```python
from build123d import *

# Parameters (mm, degrees)
CROQUIS1_R                 = 4
SALIENTE_EXTRUIR1_DEPTH    = 12.5
CROQUIS2_W                 = 30
CROQUIS2_H                 = 15
CORTAR_EXTRUIR1_DEPTH      = 52.973550966
CROQUIS3_R                 = 4
CORTAR_EXTRUIR2_DEPTH      = 52.973550966
CROQUIS4_R                 = 11.25
CORTAR_EXTRUIR3_DEPTH      = 3.5
CORTAR_EXTRUIR4_DEPTH      = 52.278650528
CORTAR_EXTRUIR4_DEPTH_BACK = 52.278650528
CROQUIS5_R                 = 5.25
CROQUIS6_R                 = 16.25
CROQUIS6_R_2               = 11.25
SALIENTE_EXTRUIR2_DEPTH    = 12
CHAFL_N1_SIZE              = 1
SKETCH1_R                  = 1.75
CUT_EXTRUDE1_DEPTH         = 10
CIRPATTERN1_COUNT          = 4


with BuildPart() as part:
    # Croquis1 → Saliente-Extruir1 (new, symmetric)
    with BuildSketch(Plane.XY):
        with BuildLine():
            Line((-43, 6), (43, 6))
            ThreePointArc((43, 6), (49, 0), (43, -6))
            Line((43, -6), (-43, -6))
            ThreePointArc((-43, -6), (-49, 0), (-43, 6))
        make_face()
        with Locations((-43, 0)):
            Circle(CROQUIS1_R, mode=Mode.SUBTRACT)
        with Locations((43, 0)):
            Circle(CROQUIS1_R, mode=Mode.SUBTRACT)
    extrude(amount=SALIENTE_EXTRUIR1_DEPTH, both=True)

    # Croquis2 → Cortar-Extruir1 (cut, through all)
    with BuildSketch(Plane(origin=(0, 6, 0), x_dir=(1, 0, 0), z_dir=(0, 1, 0))):
        with Locations((-34, 0)):
            Rectangle(CROQUIS2_W, CROQUIS2_H)
        with Locations((34, 0)):
            Rectangle(CROQUIS2_W, CROQUIS2_H)
    extrude(amount=-CORTAR_EXTRUIR1_DEPTH, mode=Mode.SUBTRACT)

    # Croquis3 → Cortar-Extruir2 (cut, through all)
    with BuildSketch(Plane(origin=(0, 6, 0), x_dir=(1, 0, 0), z_dir=(0, 1, 0))):
        with Locations(Location((0, 0, 0), (0, 0, 270))):
            Circle(CROQUIS3_R)
    extrude(amount=-CORTAR_EXTRUIR2_DEPTH, mode=Mode.SUBTRACT)

    # Croquis4 → Cortar-Extruir3 (cut)
    with BuildSketch(Plane(origin=(0, 6, 0), x_dir=(1, 0, 0), z_dir=(0, 1, 0))):
        with Locations(Location((0, 0, 0), (0, 0, 270))):
            Circle(CROQUIS4_R)
    extrude(amount=-CORTAR_EXTRUIR3_DEPTH, mode=Mode.SUBTRACT)

    # Croquis5 → Cortar-Extruir4 (cut, two sides: drawn at the far end of the back side and taken through both)
    with BuildSketch(Plane(origin=(0, 2.5, 0), x_dir=(1, 0, 0), z_dir=(0, 1, 0)).offset(-CORTAR_EXTRUIR4_DEPTH_BACK)):
        with Locations(Location((0, 0, 0), (0, 0, 270))):
            Circle(CROQUIS5_R)
    extrude(amount=CORTAR_EXTRUIR4_DEPTH + CORTAR_EXTRUIR4_DEPTH_BACK, mode=Mode.SUBTRACT)

    # Croquis6 → Saliente-Extruir2 (add)
    with BuildSketch(Plane(origin=(0, 6, 0), x_dir=(1, 0, 0), z_dir=(0, 1, 0))):
        Circle(CROQUIS6_R)
        with Locations(Location((0, 0, 0), (0, 0, 270))):
            Circle(CROQUIS6_R_2, mode=Mode.SUBTRACT)
    extrude(amount=-SALIENTE_EXTRUIR2_DEPTH)

    # Chaflán1
    chafl_n1_edges = [part.edges().sort_by_distance(p)[0] for p in [
        (0, -6, -16.25),
        (0, 6, -16.25),
        (0, 6, 16.25),
        (0, -6, 16.25),
        (49, 0, 12.5),
        (26.691639914, 6, 12.5),
        (-49, 0, -7.5),
        (-31, -6, -7.5),
        (-49, 0, 7.5),
        (-31, -6, 7.5),
        (-19, 0, 7.5),
        (-19, -6, 0),
        (-31, 6, 7.5),
        (-19, 6, 0),
        (-31, 6, -7.5),
        (-49, 0, 12.5),
        (26.691639914, 6, -12.5),
        (31, 6, 7.5),
        (31, 6, -7.5),
        (19, 6, 0),
        (49, 0, -7.5),
        (31, -6, -7.5),
        (49, 0, 7.5),
        (31, -6, 7.5),
        (49, 0, -12.5),
        (19, -6, 0),
        (-26.691639914, -6, -12.5),
        (-49, 0, -12.5),
        (-26.691639914, -6, 12.5),
        (-26.691639914, 6, 12.5),
        (-26.691639914, 6, -12.5),
        (26.691639914, -6, -12.5),
        (26.691639914, -6, 12.5),
    ]]
    chamfer(chafl_n1_edges, length=CHAFL_N1_SIZE)

    # Sketch1 → Cut-Extrude1 (cut)
    with BuildSketch(Plane(origin=(0, 2.5, 0), x_dir=(1, 0, 0), z_dir=(0, 1, 0))):
        with Locations(Location((0, 8, 0), (0, 0, 270))):
            Circle(SKETCH1_R)
    cut_extrude1 = extrude(amount=-CUT_EXTRUDE1_DEPTH, mode=Mode.SUBTRACT)

    # CirPattern1: Cut-Extrude1 ×4 about axis
    cirpattern1_axis = Axis((0, 0, 0), (0, 1, 0))
    for i in range(1, CIRPATTERN1_COUNT):
        add(cut_extrude1.rotate(cirpattern1_axis, i * 360 / CIRPATTERN1_COUNT), mode=Mode.SUBTRACT)


solid = part.part
```
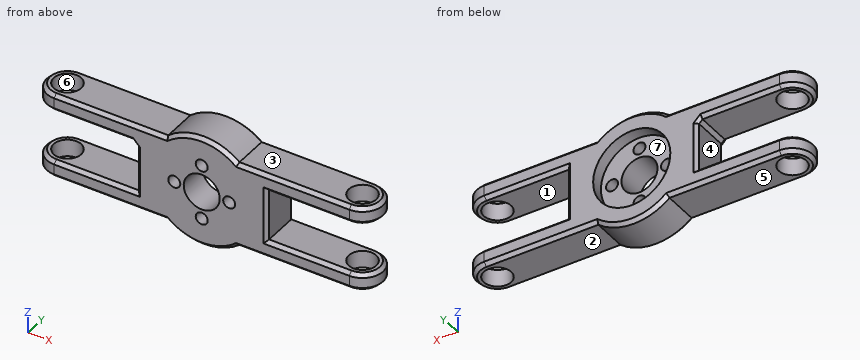
For this review, take the finished solid that the model builds, in its own axes (mm). Face numbers are marked on the shaded views. A direction names the side the tool comes from. Round coordinates to 2 decimals unless told otherwise and drop trailing zeros. Write each loop counter-clockwise with the first axis right and the second up, starting at its lowest first coordinate (ties: lowest second). Pieces come first, ordered by that corner, then holes. Notation, with made-up numbers: (-6, 30.25) - (9, 30.25) arc R5 cw to (9, 38.25) - close; hole circle Ø5 at (34.5, 21.25). An arc over 180 degrees is marked (long way). Answer as a JSON object with one key per item and string values.
1. We need section B-B on y = 0. Count the separate pieces of the cut face and the enclosed holes in it, then the cut area to 3 significant figures.
Response values:
{"separate pieces": "5", "enclosed holes": "5", "area": "1,370 mm2"}
2. For pin 1 Ø5 at (x, y) = (-34.5, 2) entering from +Z; pin 2 Ø4.5 at (x, z) = (-8, 0) entering from +Y; pin 3 Ø1.5 at (y, z) = (-0.5, 4) entering from -X, all flat-tipped, find the tip position at first contact; note any pin that passes through.
Response values:
{"pin 1": "stops at z = 12.5", "pin 2": "stops at y = 2.5", "pin 3": "stops at x = -19"}
3. We need section C-C on x = -15. Give the boundary of the cut face in (y, z), then the cut area to 3 significant figures.
Response values:
{"outline": "(-6, -11.5) - (-5, -12.5) - (5, -12.5) - (6, -11.5) - (6, 11.5) - (5, 12.5) - (-5, 12.5) - (-6, 11.5) - close", "area": "298 mm2"}
4. Tool access review of the marked faces 1, 2, 3 and 4: name each direction out of +Z, -Z, +X, -X, +Y, -Y from which nothing blocks a thin tool from reaching the whole face with its end or side.
Response values:
{"face 1": "+X, +Y, -Y", "face 2": "-Z, +X, +Y, -Y", "face 3": "+Z, +X, +Y, -Y", "face 4": "-X, +Y, -Y"}
5. Draft analysis for pull direction Y (two halves, no side actions). For the marked faces 5, 6 and 7, state which applies: +Y half, -Y half, draft (parallel to the pull), parting line (faces both ways), or undercut.
Response values:
{"face 5": "draft", "face 6": "undercut", "face 7": "+Y half"}
6. We need section A-A on x = 24. Give the boundary of the cut face in (y, z), then the cut area to 3 significant figures.
Response values:
{"outline": "(-6, -11.5) - (-5, -12.5) - (5, -12.5) - (6, -11.5) - (6, -8.5) - (5, -7.5) - (-5, -7.5) - (-6, -8.5) - close; (-6, 8.5) - (-5, 7.5) - (5, 7.5) - (6, 8.5) - (6, 11.5) - (5, 12.5) - (-5, 12.5) - (-6, 11.5) - close", "area": "116 mm2"}
7. To check wall thickness, follow line 1 along X through (y, z) = (0, -10.1); line 2 along Z through (x, y) = (-45, -3.5); line 3 along X through (y, z) = (-4, 1). State the ranges of each line that lie inside material, in increasing order.
Response values:
{"line 1": "x = -49 to -47, -39 to 39, 47 to 49", "line 2": "z = -12.5 to -7.5, 7.5 to 12.5", "line 3": "x = -19 to -9.44, -6.56 to -5.15, 5.15 to 6.56, 9.44 to 19"}
